```python
from build123d import *

# Parameters (mm, degrees)
F5_W      = 32
F5_H      = 175
F6_DEPTH  = 16
F7_W      = 21
F7_H      = 30.5
F8_DEPTH  = 32.001
F9_W      = 5.25
F9_H      = 66
F9_W_2    = 8
F9_H_2    = 4
F10_DEPTH = 18.5
F12_W     = 26
F12_H     = 78
F13_DEPTH = 10.5
F14_DEPTH = 175.001
F15_W     = 8
F15_H     = 4
F16_DEPTH = 21.501
F17_R     = 13
F18_DEPTH = 9
F19_R     = 1
F19_R_2   = 8
F20_DEPTH = 3


with BuildPart() as f6:
    # F5 (on Top) → F6 (new body, symmetric)
    with BuildSketch(Plane.XY):
        Rectangle(F5_W, F5_H)
    extrude(amount=F6_DEPTH, both=True)

    # F7 (on face) → F8 (cut, through all)
    with BuildSketch(Plane.XY.offset(16)):
        with Locations((0, 57.25)):
            Rectangle(F7_W, F7_H)
        with Locations((0, -57.25)):
            Rectangle(F7_W, F7_H)
    extrude(amount=-F8_DEPTH, mode=Mode.SUBTRACT)

    # F9 (on face) → F10 (cut)
    with BuildSketch(Plane.XY.offset(16)):
        with Locations((6.625, 0)):
            Rectangle(F9_W, F9_H)
        Rectangle(F9_W_2, F9_H)
        with Locations((-6.625, 0)):
            Rectangle(F9_W, F9_H)
        with Locations((0, 35)):
            Rectangle(F9_W_2, F9_H_2)
        with Locations((0, -35)):
            Rectangle(F9_W_2, F9_H_2)
    extrude(amount=-F10_DEPTH, mode=Mode.SUBTRACT)

    # F12 (on face) → F13 (cut)
    with BuildSketch(Plane(origin=(0, 0, -16), x_dir=(1, 0, 0), z_dir=(0, 0, -1))):
        Rectangle(F12_W, F12_H)
    extrude(amount=-F13_DEPTH, mode=Mode.SUBTRACT)

    # F11 (on face) → F14 (intersect, through all)
    with BuildSketch(Plane.XZ.offset(87.5)):
        with BuildLine():
            ThreePointArc((0, -16), (11.313708499, -11.313708499), (16, 0))
            ThreePointArc((16, 0), (11.313708499, 11.313708499), (0, 16))
            ThreePointArc((0, 16), (-11.313708499, 11.313708499), (-16, 0))
            ThreePointArc((-16, 0), (-11.313708499, -11.313708499), (0, -16))
        make_face()
    extrude(amount=-F14_DEPTH, mode=Mode.INTERSECT)

    # F15 (on face) → F16 (cut, through all)
    with BuildSketch(Plane(origin=(0, 0, -5.5), x_dir=(1, 0, 0), z_dir=(0, 0, -1))):
        with Locations((0, 35)):
            Rectangle(F15_W, F15_H)
        with Locations((0, -35)):
            Rectangle(F15_W, F15_H)
    extrude(amount=-F16_DEPTH, mode=Mode.SUBTRACT)

    # F17 (on face) → F18 (cut)
    with BuildSketch(Plane.XZ.offset(87.5)):
        Circle(F17_R)
    extrude(amount=-F18_DEPTH, mode=Mode.SUBTRACT)

    # F19 (on face) → F20 (cut)
    with BuildSketch(Plane.XZ.offset(78.5)):
        with Locations((8, -8)):
            Circle(F19_R)
        with Locations((-8, -8)):
            Circle(F19_R)
        with Locations((-8, 8)):
            Circle(F19_R)
        with Locations((8, 8)):
            Circle(F19_R)
        Circle(F19_R_2)
    extrude(amount=-F20_DEPTH, mode=Mode.SUBTRACT)


solid = f6.part
```
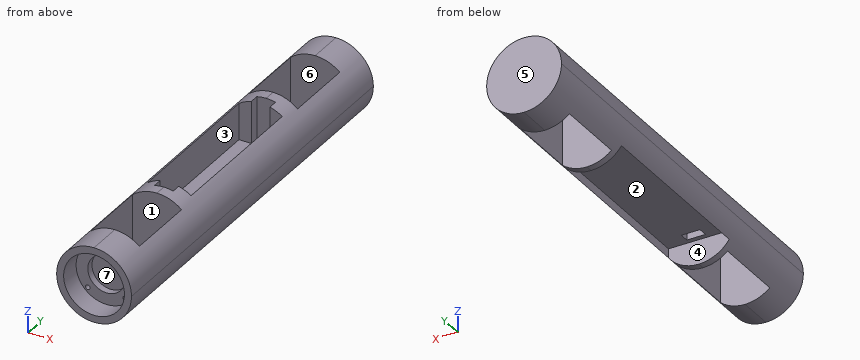
The model under review builds one solid part; all positions refer to its coordinate system, in mm. Face numbers are marked on the shaded views. A direction names the side the tool comes from. Round coordinates to 2 decimals unless told otherwise and drop trailing zeros. Write each loop counter-clockwise with the first axis right and the second up, starting at its lowest first coordinate (ties: lowest second). Pieces come first, ordered by that corner, then holes. Notation, with made-up numbers: (47, 6.25) - (103, 6.25) arc R15 ccw to (103, 16.25) - close; hole circle Ø7 at (-24, 28). An arc over 180 degrees is marked (long way). Answer as CSV lines item,"result". Start each with the question number.
(1) For the marked faces 1, 2 and 3, list the 3-axis set-ups (+Z, -Z, +X, -X, +Y, -Y) from which the entire face can be reached by the end or side of a thin tool; tool diameter is ignored.
(2) We need section A-A on y = 67.5. State the section outline as (x, z) points.
(3) We need section C-C on y = -8. State the section outline as (x, z) points, plus the area to 3 significant figures.
(4) To check wall thickness, follow line 1 (Y direction, x = -0.5, z = -1); line 2 (Y direction, x = 2.5, z = 13.5); line 3 (X direction, y = -44, z = -10.5). State the ranges of each line that lie inside material, in increasing order.
(5) We need section D-D on y = -74. State the section outline as (x, z) points.
(6) For pin 1 Ø3 at (y, z) = (64.5, 4.5) entering from +X; pin 2 Ø1.1 at (y, z) = (12.5, -6.5) entering from -X; pin 3 Ø2 at (y, z) = (59, -5) entering from +X, all flat-tipped, find the tip position at first contact; note any pin that passes through.
(7) Draft analysis for pull direction Y (two halves, no side actions). For the marked faces 4, 5, 6 and 7, state which applies: pulls with the +Y half, pulls with the -Y half, needs draft (parallel to the pull), parting line crosses it, or undercut.
(8) We need section B-B on z = 1.5. Give the number of separate pieces and of enclosed holes in the cut face, plus the area to 3 significant figures.
Worked answers:
1,face 1,"+Z, -Z"
1,face 2,"-Z"
1,face 3,"+Z"
2,outline,"(-10.5, -12.07) - (-10.5, 12.07) arc R16 ccw to start; (10.5, -12.07) arc R16 ccw to (10.5, 12.07) - close"
3,outline,"(-13, -9.33) - (-13, -5.5) - (13, -5.5) - (13, -9.33) arc R16 ccw to (9.25, 13.06) - (9.25, -2.5) - (-9.25, -2.5) - (-9.25, 13.06) arc R16 ccw to start"
3,area,"258 mm²"
4,line 1,"-75.5 to -72.5, -42 to -37, 37 to 42, 72.5 to 87.5"
4,line 2,"-87.5 to -72.5, -42 to -37, 37 to 42, 72.5 to 87.5"
4,line 3,"-12.07 to -10.5, 10.5 to 12.07"
5,outline,"circle Ø32 at (0, 0)"
6,pin 1,"x = 15.72"
6,pin 2,"x = -14.85"
6,pin 3,"x = 15.49"
7,face 4,"undercut"
7,face 5,"pulls with the +Y half"
7,face 6,"undercut"
7,face 7,"pulls with the -Y half"
8,separate pieces,"1"
8,enclosed holes,"3"
8,area,"2,730 mm²"
